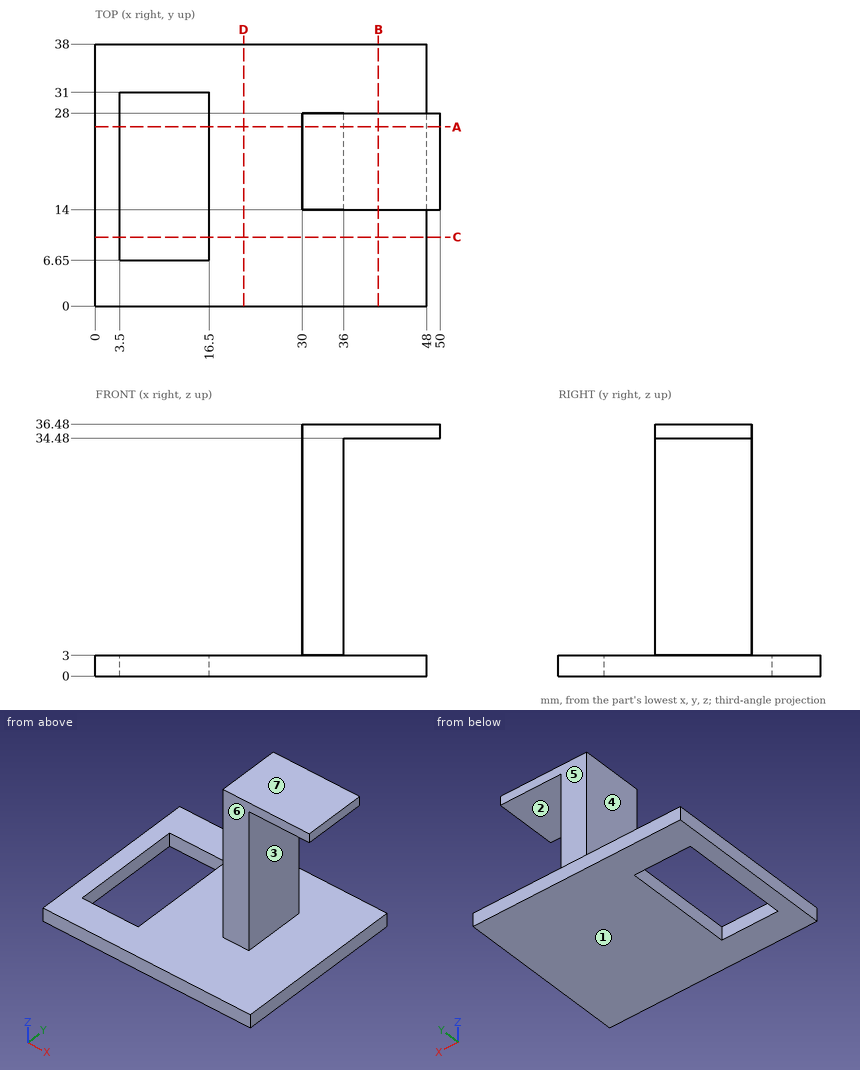
Print and shaded views of the part. All mm, measured from the part's lowest x, y and z. A direction names the side the tool comes from. Give positions to 0.01 mm unless a question says otherwise; leave off trailing zeros. Order: outer loops, then holes, each group sorted by start corner. A loop starts at its lowest first (then second) coordinate and runs counter-clockwise, first axis right, second up. Notation, with made-up numbers: (43.5, 45) - (78.5, 45) arc R6 ccw to (78.5, 56) - close; hole circle Ø10 at (49.25, 29.5). An arc over 180 degrees is marked (long way). One line per item, written item: value.
Item 1: Slice it at C-C (y = 10). List the corners of the cut face in (x, z).
Response values:
outline: (0, 0) - (3.5, 0) - (3.5, 3) - (0, 3) - close; (16.5, 0) - (48, 0) - (48, 3) - (16.5, 3) - close
Item 2: Two-plate mould, pull along Z, no slides. Class the marked faces 1, 2, 3 and 4: released by +Z, released by -Z, zero draft, split by the parting line, or undercut.
Response values:
face 1: released by -Z
face 2: undercut
face 3: undercut
face 4: zero draft
Item 3: Slice it at D-D (x = 21.5). List the corners of the cut face in (y, z).
Response values:
outline: (0, 0) - (38, 0) - (38, 3) - (0, 3) - close
Item 4: Pin check, flat tips, straight feed: pin 1 Ø12 at (y, z) = (16.5, 27.5) entering from +X; pin 2 Ø2 at (x, y) = (20.5, 14.5) entering from +Z; pin 3 Ø1.5 at (y, z) = (26, 1) entering from +X. Stop position of each tip, or through.
Response values:
pin 1: x = 36
pin 2: z = 3
pin 3: x = 48
Item 5: Tool access for the marked faces 5, 6 and 7: list every direction of +Z, -Z, +X, -X, +Y, -Y with a clear straight run to the whole face (end or side of a thin tool).
Response values:
face 5: +Z, +X, -X, +Y
face 6: +Z, +X, -X, -Y
face 7: +Z, +X, -X, +Y, -Y
Item 6: Wall check: line 1 (Z direction, x = 44, y = 18.5); line 2 (Z direction, x = 21.5, y = 13); line 3 (X direction, y = 18.5, z = 22). Give the ranges that are in metal, low to high.
Response values:
line 1: 0 to 3, 34.48 to 36.48
line 2: 0 to 3
line 3: 30 to 36
Item 7: Slice it at B-B (x = 41). List the corners of the cut face in (y, z), then the cut area to 3 significant figures.
Response values:
outline: (0, 0) - (38, 0) - (38, 3) - (0, 3) - close; (14, 34.48) - (28, 34.48) - (28, 36.48) - (14, 36.48) - close
area: 142 mm2
Item 8: Slice it at A-A (y = 26). List the corners of the cut face in (x, z), then the cut area to 3 significant figures.
Response values:
outline: (0, 0) - (3.5, 0) - (3.5, 3) - (0, 3) - close; (16.5, 0) - (48, 0) - (48, 3) - (36, 3) - (36, 34.48) - (50, 34.48) - (50, 36.48) - (30, 36.48) - (30, 3) - (16.5, 3) - close
area: 334 mm2
